Design review of the part built by this model. Coordinates are the model's own, in mm. Give positions to 0.01 mm unless a question says otherwise; leave off trailing zeros. Loops run counter-clockwise (first coordinate to the right, second up) from the corner with the lowest first, then second, coordinate; pieces in that order, holes last. Notation, with made-up numbers: (-24, 1.25) -> (4, 1.25) arc R16 ccw to (4, 28.25) -> close; hole circle Ø10 at (69, 11.5). An arc over 180 degrees is marked (long way). Use a Markdown table: item, result. Add a question column.
1. Add section C-C (y = 35). State the section outline as (x, z) points (3 decimals), and give its area (3 significant figures).
2. Add section A-A (y = 0). State the section outline as (x, z) points (1 decimal).
3. Add section B-B (z = 0). State the section outline as (x, y) points (3 decimals).
4. To check wall thickness, follow line 1 (Z direction, x = 2.25, y = -100) (1 decimal); line 2 (Y direction, x = 1.55, z = 2); line 3 (Z direction, x = 1.8, y = -53) (3 decimals). State the ranges of each line that lie inside material, in increasing order.
5. For pin 1 Ø3 at (y, z) = (0, -13.47) entering from -X; pin 2 Ø1 at (x, z) = (1, -1.5) entering from +Y, all flat-tipped, find the tip position at first contact; note any pin that passes through.
6. Add section D-D (x = 1.5). Count the separate pieces of the cut face and the enclosed holes in it, and give its area (3 significant figures).
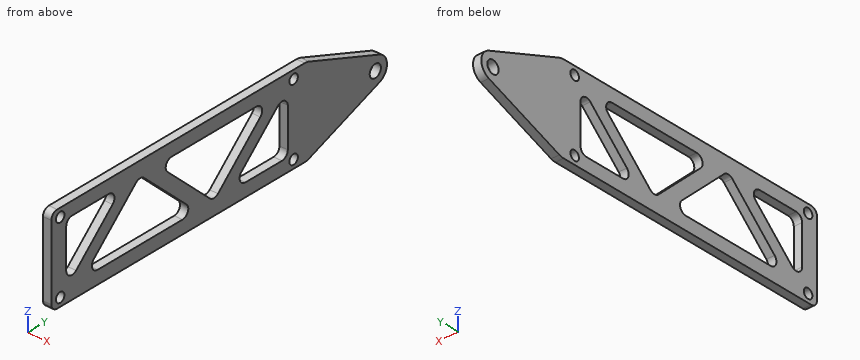
```python
from build123d import *

# Parameters (mm, degrees)
SKETCH1_W           = 41.514809608
SKETCH1_H           = 98.81
SKETCH1_R           = 1.8288
SKETCH1_R_2         = 2.413
BOSS_EXTRUDE1_DEPTH = 3.175
SKETCH2_W           = 4.112404804
SKETCH2_H           = 141.223
CUT_EXTRUDE1_DEPTH  = 106.912542124
FILLET1_R           = 2.5
FILLET2_R           = 5


with BuildPart() as part:
    # Sketch1 → Boss-Extrude1 (new body)
    # profile 1 of 2: a face of its own
    with BuildSketch(Plane(origin=(0, 0, 0), x_dir=(0, 0, -1), z_dir=(1, 0, 0))):
        with Locations((0, -54.405)):
            Rectangle(SKETCH1_W, SKETCH1_H)
        with Locations((13.4747, -100)):
            Circle(SKETCH1_R, mode=Mode.SUBTRACT)
        with Locations((-13.4747, -100)):
            Circle(SKETCH1_R, mode=Mode.SUBTRACT)
    # profile 2 of 2: a face of its own
    with BuildSketch(Plane(origin=(0, 0, 0), x_dir=(0, 0, -1), z_dir=(1, 0, 0))):
        Polygon((0, 48.916537522), (20.757404804, -5), (-20.757404804, -5), align=None)
        with Locations((13.4747, 0)):
            Circle(SKETCH1_R, mode=Mode.SUBTRACT)
        with Locations((0, 35)):
            Circle(SKETCH1_R_2, mode=Mode.SUBTRACT)
        with Locations((-13.4747, 0)):
            Circle(SKETCH1_R, mode=Mode.SUBTRACT)
    extrude(amount=BOSS_EXTRUDE1_DEPTH)

    # Sketch2 → Cut-Extrude1 (cut, through all)
    with BuildSketch(Plane(origin=(3.175, 0, 0), x_dir=(0, 0, -1), z_dir=(1, 0, 0))):
        Polygon((11.645, -2.5), (-11.645, -2.5), (11.645, -26.898674048), align=None)
        Polygon((-11.645, -9.741325952), (11.645, -34.14), (-11.645, -58.538674048), (-11.645, -34.14), align=None)
        Polygon((-11.645, -73.021325952), (-11.645, -97.42), (11.645, -97.42), align=None)
        Polygon((11.645, -41.381325952), (11.645, -65.78), (11.645, -90.178674048), (-11.645, -65.78), align=None)
        with Locations((-18.701202402, -33.1985)):
            Rectangle(SKETCH2_W, SKETCH2_H)
        with Locations((18.701202402, -33.1985)):
            Rectangle(SKETCH2_W, SKETCH2_H)
    extrude(amount=-CUT_EXTRUDE1_DEPTH, mode=Mode.SUBTRACT)

    # Fillet1
    fillet1_edges = [part.edges().sort_by_distance(p)[0] for p in [
        (1.5875, -103.81, -16.645),
        (1.5875, -9.741325952, 11.645),
        (1.5875, -34.14, -11.645),
        (1.5875, -58.538674048, 11.645),
        (1.5875, -26.898674048, -11.645),
        (1.5875, -2.5, 11.645),
        (1.5875, -2.5, -11.645),
        (1.5875, -90.178674048, -11.645),
        (1.5875, -65.78, 11.645),
        (1.5875, -41.381325952, -11.645),
        (1.5875, -103.81, 16.645),
        (1.5875, -73.021325952, 11.645),
        (1.5875, -97.42, -11.645),
        (1.5875, -97.42, 11.645),
    ]]
    fillet(fillet1_edges, radius=FILLET1_R)

    # Fillet2
    fillet2_edges = [part.edges().sort_by_distance(p)[0] for p in [
        (1.5875, 48.916537522, 0),
        (1.5875, 5.681808734, -16.645),
        (1.5875, 5.681808734, 16.645),
    ]]
    fillet(fillet2_edges, radius=FILLET2_R)


solid = part.part
```
Taken from the geometry:
| question | item | result |
|---|---|---|
| 1 | outline | (0, -5.358) -> (3.175, -5.358) -> (3.175, -2.413) -> (0, -2.413) -> close; (0, 2.413) -> (3.175, 2.413) -> (3.175, 5.358) -> (0, 5.358) -> close |
| 1 | area | 18.7 mm^2 |
| 2 | outline | (0, -16.6) -> (3.2, -16.6) -> (3.2, -15.3) -> (0, -15.3) -> close; (0, -11.6) -> (3.2, -11.6) -> (3.2, 11.6) -> (0, 11.6) -> close; (0, 15.3) -> (3.2, 15.3) -> (3.2, 16.6) -> (0, 16.6) -> close |
| 3 | outline | (0, -103.81) -> (3.175, -103.81) -> (3.175, -97.42) -> (0, -97.42) -> close; (0, -85.221) -> (3.175, -85.221) -> (3.175, -77.979) -> (0, -77.979) -> close; (0, -53.581) -> (3.175, -53.581) -> (3.175, -46.339) -> (0, -46.339) -> close; (0, -21.941) -> (3.175, -21.941) -> (3.175, -14.699) -> (0, -14.699) -> close; (0, -2.5) -> (3.175, -2.5) -> (3.175, 32.587) -> (0, 32.587) -> close; (0, 37.413) -> (3.175, 37.413) -> (3.175, 40) -> (0, 40) -> close |
| 4 | line 1 | z = -16.6 to -15.3, -11.6 to 11.6, 15.3 to 16.6 |
| 4 | line 2 | y = -103.81 to -97.42, -83.13 to -75.88, -55.68 to -48.43, -19.85 to -12.6, -2.5 to 33.65, 36.35 to 39.58 |
| 4 | line 3 | z = -16.645 to -11.645, -0.554 to 6.358, 11.545 to 16.645 |
| 5 | pin 1 | passes through |
| 5 | pin 2 | stops at y = 39.9 |
| 6 | separate pieces | 1 |
| 6 | enclosed holes | 9 |
| 6 | area | 2,630 mm^2 |
